Read the model definition and answer for the solid it produces. Units are mm, in the model's axes. A direction names the side the tool comes from. Coordinates: 2 decimals unless noted, no trailing zeros. Write each loop counter-clockwise with the first axis right and the second up, starting at its lowest first coordinate (ties: lowest second). Pieces come first, ordered by that corner, then holes.
1) Find the intervals of material crossed by line 1 (Z direction, x = 9, y = 32.5); line 2 (X direction, y = 30.5, z = -6.25); line 3 (Z direction, x = -1, y = 11.5), in increasing order.
2) Which of the six approach directions +Z, -Z, +X, -X, +Y, -Y give full straight-line access (tool end or side, diameter ignored) to faces 1 (the face through (-3.604, 37.867, 11.446)), 2 (the face through (8, 30, 5))?
3) Each of these flat-tipped pins is pushed along its axis until it touches: pin 1 Ø2 at (x, y) = (-5, 21.5) entering from +Z; pin 2 Ø2 at (x, z) = (7.5, 2) entering from +Y; pin 3 Ø10 at (x, y) = (7.5, 7.5) entering from +Z. Where does it stop, or does it pass through?
4) The part is cut by section C-C (y = 19). Determine the outline of the cut face in (x, z).
from build123d import *

# Parameters (mm, degrees)
CHAMFER_1_SIZE = 1.5


with BuildPart() as part:
    # 草图1 → 旋转1 (revolve)
    with BuildSketch(Plane.XY, mode=Mode.PRIVATE) as revolve_1_sk:
        with BuildLine():
            Line((0, 0), (-7.85, 0))
            Line((-7.85, 0), (-7.85, 22))
            Line((-7.85, 22), (-8.85, 22))
            Line((-8.85, 22), (-8.85, 30))
            Line((-8.85, 30), (-10.5, 30))
            Line((-10.5, 30), (-10.5, 35))
            Line((-10.5, 35), (-12, 35))
            Line((-12, 35), (-12, 39.196412484))
            ThreePointArc((-12, 39.196412484), (-6.013438137, 39.798878399), (0, 40))
            Line((0, 40), (0, 0))
        make_face()
    revolve(revolve_1_sk.sketch.rotate(Axis((0, 40, 0), (0, -1, 0)), 270), axis=Axis((0, 40, 0), (0, -1, 0)))

    # 倒角1
    chamfer_1_edges = [part.edges().sort_by_distance(p)[0] for p in [
        (0, 35, -12),
    ]]
    chamfer(chamfer_1_edges, length=CHAMFER_1_SIZE - 0.0001)  # a hair under: the kernel refuses the full size


solid = part.part
Reported:
1. line 1: z = -5.41 to 5.41
1. line 2: x = -8.44 to 8.44
1. line 3: z = -7.79 to 7.79
2. face 1: +Y, -Y
2. face 2: -Y
3. pin 1: stops at z = 7.83
3. pin 2: stops at y = 39.75
3. pin 3: stops at z = 7.44
4. outline: circle Ø15.7 at (0, 0)
